Geometry check sheet. Reference: drawing and pictorial views, mm from the part's lowest x, y, z. A direction names the side the tool comes from. Round coordinates to 2 decimals unless told otherwise and drop trailing zeros. Write each loop counter-clockwise with the first axis right and the second up, starting at its lowest first coordinate (ties: lowest second). Pieces come first, ordered by that corner, then holes. Notation, with made-up numbers: M 19.25,-17.5 L 48.25,-17.5 A11 cw 48.25,-13.5 Z; hole C 55.5,77 d7. An arc over 180 degrees is marked long. Answer in a Markdown table with one row per item. Add a question column.
1. Material ranges on probe 1 along Y at (x, z) = (16.51, 7.75); probe 2 along Y at (x, z) = (16.51, 16.9); probe 3 along Z at (x, y) = (14.5, 6.5) (3 decimals), recorded low to high.
2. Sectioned sample at D-D on z = 6.25. Record the cut outline in (x, y).
3. Draft check along X on the marked faces 3, 4 and 5. Enter one of: pulls with the +X half, pulls with the -X half, needs draft (parallel to the pull), parting line crosses it, or undercut.
4. Sectioned sample at C-C on z = 17.25. Record the cut outline in (x, y), plus the area to 3 significant figures.
5. Go/stop test with flat-tipped pins: pin 1 Ø3 at (x, z) = (16, 8) entering from +Y; pin 2 Ø1 at (x, z) = (28.5, 15) entering from +Y; pin 3 Ø1.5 at (x, y) = (4.5, 27) entering from -Z; pin 4 Ø1.5 at (y, z) = (5, 8.5) entering from +X. Record where each tip stops, or that it passes through.
6. Set-up check for the marked faces 1 and 2: record each of +Z, -Z, +X, -X, +Y, -Y from which the full face is reachable in a straight line by a thin tool's end or side.
7. Sectioned sample at B-B on y = 16.51. Record the cut outline in (x, z) (3 decimals), plus the area to 3 significant figures.
8. Sectioned sample at A-A on x = 16.51. Record the cut outline in (y, z) (3 decimals), plus the area to 3 significant figures.
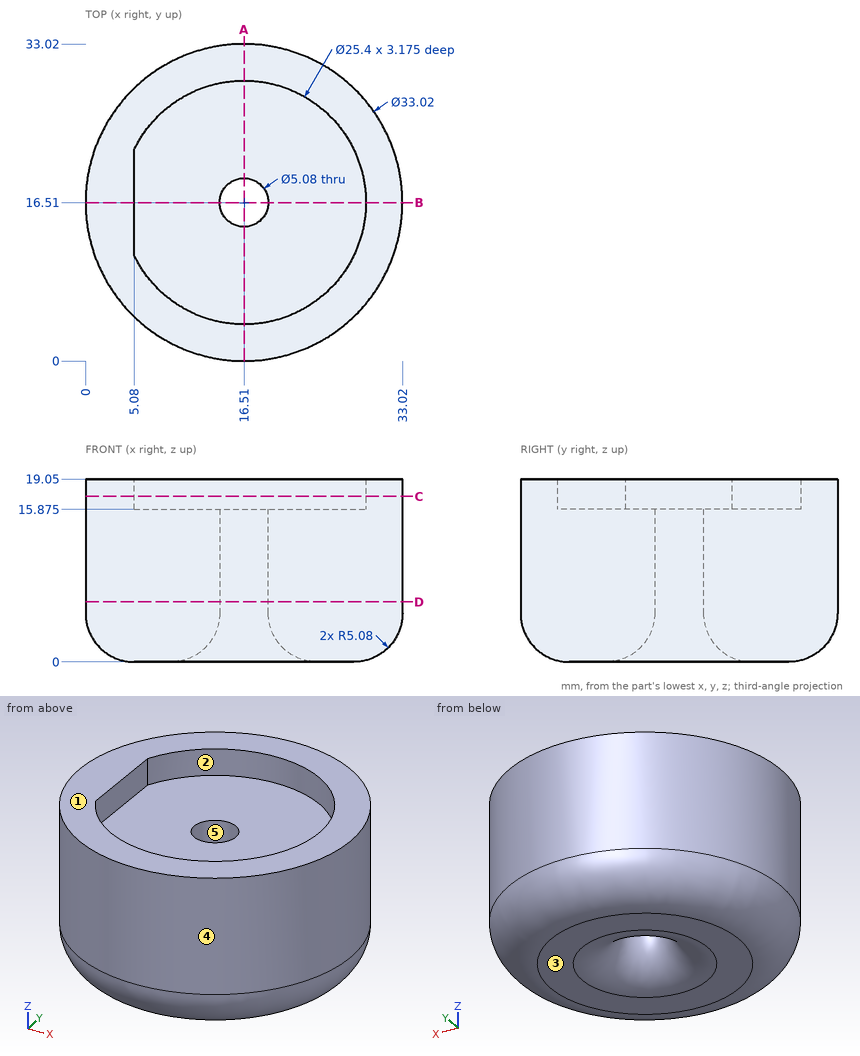
Geometry check:
| question | item | result |
|---|---|---|
| 1 | probe 1 | y = 0 to 13.97, 19.05 to 33.02 |
| 1 | probe 2 | y = 0 to 3.81, 29.21 to 33.02 |
| 1 | probe 3 | z = 0 to 15.875 |
| 2 | outline | C 16.51,16.51 d33.02; hole C 16.51,16.51 d5.08 |
| 3 | face 3 | needs draft |
| 3 | face 4 | parting line crosses it |
| 3 | face 5 | undercut |
| 4 | outline | C 16.51,16.51 d33.02; hole M 5.08,10.97 A12.7 ccw long 5.08,22.05 Z |
| 4 | area | 359 mm2 |
| 5 | pin 1 | stops at y = 33.02 |
| 5 | pin 2 | stops at y = 28.37 |
| 5 | pin 3 | stops at z = 1.67 |
| 5 | pin 4 | stops at x = 29.03 |
| 6 | face 1 | +Z, +X, -X, +Y, -Y |
| 6 | face 2 | +Z |
| 7 | outline | M 0,5.08 A5.08 ccw 5.08,0 L 8.89,0 A5.08 ccw 13.97,5.08 L 13.97,15.875 L 5.08,15.875 L 5.08,19.05 L 0,19.05 Z; M 19.05,5.08 A5.08 ccw 24.13,0 L 27.94,0 A5.08 ccw 33.02,5.08 L 33.02,19.05 L 29.21,19.05 L 29.21,15.875 L 19.05,15.875 Z |
| 7 | area | 450 mm2 |
| 8 | outline | M 0,5.08 A5.08 ccw 5.08,0 L 8.89,0 A5.08 ccw 13.97,5.08 L 13.97,15.875 L 3.81,15.875 L 3.81,19.05 L 0,19.05 Z; M 19.05,5.08 A5.08 ccw 24.13,0 L 27.94,0 A5.08 ccw 33.02,5.08 L 33.02,19.05 L 29.21,19.05 L 29.21,15.875 L 19.05,15.875 Z |
| 8 | area | 446 mm2 |
